```python
from build123d import *

# Parameters (mm, degrees)
SKETCH1_W                       = 15.1
SKETCH1_H                       = 46.4
SKETCH1_W_2                     = 9.1
SKETCH1_H_2                     = 40.4
BOSS_EXTRUDE1_DEPTH             = 4
TAP_DRILL_FOR_M2X0_4_TAP1_D     = 1.8
TAP_DRILL_FOR_M2X0_4_TAP1_DEPTH = 10
TAP_DRILL_FOR_M2X0_4_TAP1_TIP   = 0.540774557
BOSS_EXTRUDE2_DEPTH             = 46.4


with BuildPart() as part:
    # Sketch1 → Boss-Extrude1 (new body)
    # profile 1 of 2: a face of its own
    with BuildSketch(Plane.XY):
        Rectangle(SKETCH1_W, SKETCH1_H)
        Rectangle(SKETCH1_W_2, SKETCH1_H_2, mode=Mode.SUBTRACT)
    # profile 2 of 2: a face of its own
    with BuildSketch(Plane.XY):
        Rectangle(SKETCH1_W_2, SKETCH1_H_2)
    extrude(amount=BOSS_EXTRUDE1_DEPTH)

    # Tap Drill for M2x0.4 Tap1
    with Locations(Plane(origin=(-4.55, 20.2, 4), x_dir=(1, 0, 0), z_dir=(0, 0, 1))):
        with Locations((0, 0), (9.1, 0), (9.1, -40.4), (0, -40.4)):
            Hole(TAP_DRILL_FOR_M2X0_4_TAP1_D / 2, depth=TAP_DRILL_FOR_M2X0_4_TAP1_DEPTH)
            with Locations((0, 0, -(TAP_DRILL_FOR_M2X0_4_TAP1_DEPTH + TAP_DRILL_FOR_M2X0_4_TAP1_TIP / 2))):  # 118° drill point
                Cone(0, TAP_DRILL_FOR_M2X0_4_TAP1_D / 2, TAP_DRILL_FOR_M2X0_4_TAP1_TIP, mode=Mode.SUBTRACT)

    # Sketch5 → Boss-Extrude2 (add)
    with BuildSketch(Plane(origin=(0, -23.2, 0), x_dir=(-1, 0, 0), z_dir=(0, -1, 0))):
        Polygon((-7.55, -4), (7.55, -8.046032806), (7.55, -4), align=None)
    extrude(amount=-BOSS_EXTRUDE2_DEPTH)


solid = part.part
```
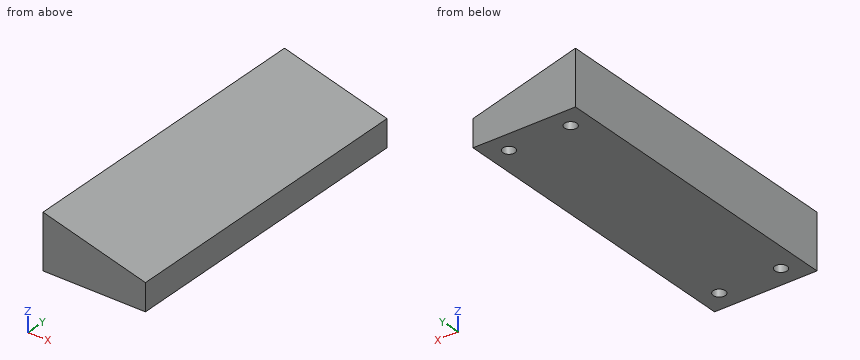
Geometry check sheet. Reference: the model listing, model coordinates, mm. Round coordinates to 2 decimals unless told otherwise and drop trailing zeros. Order: outer loops, then holes, each group sorted by start corner. A loop starts at its lowest first (then second) coordinate and runs counter-clockwise, first axis right, second up. Notation, with made-up numbers: M 7,4 L 56,4 A23 cw 56,16 Z; hole C 18.25,-3 d7. An arc over 180 degrees is marked long. Write item = value, one per line.
Q1. Section check B-B (x = -4.55). Enter the section's corners in (y, z).
Answer block:
outline = M -23.2,0 L -21.1,0 L -21.1,4 L -19.3,4 L -19.3,0 L 19.3,0 L 19.3,4 L 21.1,4 L 21.1,0 L 23.2,0 L 23.2,7.24 L -23.2,7.24 Z
Q2. Section check C-C (z = 7.25). Enter the section's corners in (x, y), plus the area to 3 significant figures.
Answer block:
outline = M -7.55,-23.2 L -4.58,-23.2 L -4.58,23.2 L -7.55,23.2 Z
area = 138 mm^2
Q3. Scan lines: line 1 (Y direction, x = -4.55, z = 1.15); line 2 (X direction, y = -19.5, z = 2.5); line 3 (Z direction, x = 6.5, y = 19). Record each from-to range of solid material in increasing order.
Answer block:
line_1 = -23.2 to -21.1, -19.3 to 19.3, 21.1 to 23.2
line_2 = -7.55 to -5.12, -3.98 to 3.98, 5.12 to 7.55
line_3 = 0 to 4.28
Q4. Section check A-A (y = -20.2). Enter the section's corners in (x, z), plus the area to 3 significant figures.
Answer block:
outline = M -7.55,0 L -5.45,0 L -5.45,4 L -3.65,4 L -3.65,0 L 3.65,0 L 3.65,4 L 5.45,4 L 5.45,0 L 7.55,0 L 7.55,4 L -7.55,8.05 Z
area = 76.5 mm^2
Q5. Depth check by flat-ended pin: pin 1 Ø1.1 at (x, y) = (-4.55, 20.2) entering from +Z; pin 2 Ø1.1 at (x, y) = (-4.55, -20.2) entering from -Z; pin 3 Ø1.5 at (x, y) = (1.5, -14.5) entering from -Z; pin 4 Ø5 at (x, y) = (2, -18) entering from +Z. Enter the tip coordinate at first touch or a pass-through.
Answer block:
pin_1 = 7.39
pin_2 = 4
pin_3 = 0
pin_4 = 6.16
Q6. Section check D-D (y = -10.5). Enter the section's corners in (x, z), plus the area to 3 significant figures.
Answer block:
outline = M -7.55,0 L 7.55,0 L 7.55,4 L -7.55,8.05 Z
area = 90.9 mm^2
